For this review, take the finished solid that the model builds, in its own axes (mm). Round coordinates to 2 decimals unless told otherwise and drop trailing zeros. Order: outer loops, then holes, each group sorted by start corner. A loop starts at its lowest first (then second) coordinate and runs counter-clockwise, first axis right, second up. Notation, with made-up numbers: M 72.5,-5.75 L 115.5,-5.75 A21 ccw 115.5,4.25 Z; hole C 33,60 d1. An arc over 180 degrees is marked long. Use a Markdown table: item, result.
from build123d import *

# Parameters (mm, degrees)
BASE_FLANGE1_DEPTH = 211
SKETCH2_R          = 1.75
EXTRUDE1_DEPTH     = 0.5


# Sheet-metal steps are written as plain solids
with BuildPart() as part:
    # Sketch1 → Base-Flange1 (new, symmetric)
    with BuildSketch(Plane.XY):
        with BuildLine():
            Line((0, 0), (-18, 0))
            ThreePointArc((-18, 0), (-23.291502622, -2), (-25.937253933, -7))
            Line((-25.937253933, -7), (-26.312253933, -9.976470225))
            Line((-26.312253933, -9.976470225), (-26.808332304, -9.913970225))
            Line((-26.808332304, -9.913970225), (-26.433332304, -6.9375))
            ThreePointArc((-26.433332304, -6.9375), (-23.622221536, -1.625), (-18, 0.5))
            Line((-18, 0.5), (0, 0.5))
            Line((0, 0.5), (0, 0))
        make_face()
    extrude(amount=BASE_FLANGE1_DEPTH, both=True)

    # Sketch2 → Extrude1 (cut)
    with BuildSketch(Plane(origin=(0, 0.5, 0), x_dir=(1, 0, 0), z_dir=(0, 1, 0))):
        with Locations(Location((-5, -196, 0), (0, 0, 180))):
            Circle(SKETCH2_R)
        with Locations((-5, 196)):
            Circle(SKETCH2_R)
        with Locations(Location((-5, 0, 0), (0, 0, 180))):
            Circle(SKETCH2_R)
    extrude(amount=-EXTRUDE1_DEPTH, mode=Mode.SUBTRACT)


solid = part.part
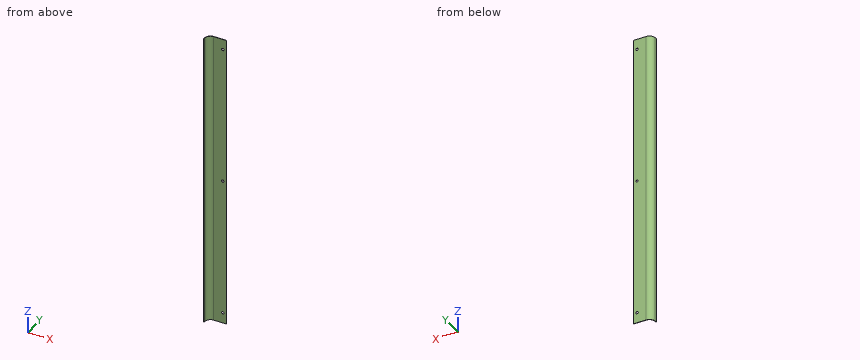
Q1. Add section A-A (z = -9). Write out the cut boundary in (x, y).
Determined:
| item | result |
|---|---|
| outline | M -26.81,-9.91 L -26.31,-9.98 L -25.94,-7 A8 cw -18,0 L 0,0 L 0,0.5 L -18,0.5 A8.5 ccw -26.43,-6.94 Z |
Q2. Add section C-C (y = -2.75). Write out the cut boundary in (x, z).
Determined:
| item | result |
|---|---|
| outline | M -24.68,-211 L -24.04,-211 L -24.04,211 L -24.68,211 Z |
Q3. Add section B-B (x = -14.5). Write out the cut boundary in (y, z), then the cut area to 3 significant figures.
Determined:
| item | result |
|---|---|
| outline | M 0,-211 L 0.5,-211 L 0.5,211 L 0,211 Z |
| area | 211 mm^2 |
Q4. Wall thickness on line 1 along Z through (x, y) = (-5, 0.35); line 2 along Y through (x, z) = (-15.75, 27.5); line 3 along X through (y, z) = (-7.25, 182): over which ranges is each line inside the solid? List them lowest first. Write a range as [from, to].
Determined:
| item | result |
|---|---|
| line 1 | z = [-211, -197.75], [-194.25, -1.75], [1.75, 194.25], [197.75, 211] |
| line 2 | y = [0, 0.5] |
| line 3 | x = [-26.47, -25.97] |
Q5. Clearance check with flat-ended pins moving along their axes: pin 1 (2 mm diameter, centred on x = -5, z = -196, fed in from -Y); pin 2 (1.5 mm diameter, centred on y = -3, z = 97, fed in from +X); pin 3 (4 mm diameter, centred on x = -5, z = 196, fed in from -Y); pin 4 (12 mm diameter, centred on x = -17, z = 167.5, fed in from -Y) (3 decimals). State where each tip first meets the part, or that it passes through.
Determined:
| item | result |
|---|---|
| pin 1 | passes through |
| pin 2 | stops at x = -23.56 |
| pin 3 | stops at y = 0 |
| pin 4 | stops at y = -1.755 |
